Check sheet for the modelled part. Datum: model origin and axes. Units: mm. Coordinates: 2 decimals unless noted, no trailing zeros. Loops run counter-clockwise (first coordinate to the right, second up) from the corner with the lowest first, then second, coordinate; pieces in that order, holes last.
Autodesk Inventor part; units mm, degrees
ref_plane "YZ Plane" through (0, 0, 0) normal (1, 0, 0) x (0, 1, 0)
ref_plane "XZ Plane" through (0, 0, 0) normal (0, 1, 0) x (-1, 0, 0)
ref_plane "XY Plane" through (0, 0, 0) normal (0, 0, 1) x (1, 0, 0)
sketch "Sketch2" plane through (0, 0, 0) normal (0, 1, 0) x (-1, 0, 0)
  line L0 (330, 50) -> (-330, 50)
  line L1 (-330, 50) -> (-330, 0)
  line L2 (-330, 0) -> (330, 0)
  line L3 (330, 0) -> (330, 50)
  circle A0 centre (-330, 0) radius 22.5
  circle A1 centre (330, 0) radius 22.5
  point P0 (0, 0)
  point P1 (0, 0)
  point P2 (-330, 22.5)
  point P3 (-307.5, 0)
  point P4 (307.5, 0)
  point P5 (330, 22.5)
  dimension "d18" = 660
  dimension "d19" = 50
  dimension "d20" = 45
extrude "Plate2" add sketch "Sketch2" along normal blind 3 contours L3 A1 L2 A0 L1 L0
equation "\"d21\" = Thickness"
equation "\"BendReliefWidth\" = Thickness"
equation "\"BendReliefDepth\" = 0.5 * Thickness"
equation "\"CornerReliefSize\" = 4 * Thickness"
equation "\"MinimumRemnant\" = 2 * Thickness"
equation "\"TransitionRadius\" = BendRadius"
equation "\"JacobiRadiusSize\" = BendRadius"
equation "\"GapSize\" = Thickness"
properties part number "MSC 0562 rib cone" material "Stainless Steel"
1) Section check B-B on z = 8. Enter the section's corners in (x, y).
Answer sheet:
outline: (-308.97, 0) - (308.97, 0) - (308.97, 3) - (-308.97, 3) - close
2) Scan lines: line 1 (X direction, y = 2.25, z = 16); line 2 (X direction, y = 0.5, z = 6.5). Record each from-to range of solid material in increasing order.
Answer sheet:
line 1: x = -314.18 to 314.18
line 2: x = -308.46 to 308.46
3) Section check A-A on y = 0.7. Enter the section's corners in (x, z), plus the area to 3 significant figures.
Answer sheet:
outline: (-330, 22.5) arc R22.5 cw to (-307.5, 0) - (307.5, 0) arc R22.5 cw to (330, 22.5) - (330, 50) - (-330, 50) - close
area: 32,200 mm2
4) Mould release check, pull along Z, two halves, no side actions. Record for faces 1 (the cylindrical face through (-313.916, 1.479, 15.734)), 2 (the flat face through (5, 0, 25)): +Z half, -Z half, draft (parallel to the pull), parting line (faces both ways), or undercut.
Answer sheet:
face 1: -Z half
face 2: draft
